```python
from build123d import *

# Parameters (mm, degrees)
F0_W     = 62
F0_H     = 82
F0_R     = 9.1
F1_DEPTH = 2
F2_R     = 10
F3_R     = 10
F4_R     = 10
F5_R     = 10
F7_DEPTH = 1


with BuildPart() as f1:
    # F0 (on Right) → F1 (new body)
    with BuildSketch(Plane.YZ):
        with Locations((0, -10)):
            Rectangle(F0_W, F0_H)
        with Locations((-20, -40)):
            Circle(F0_R, mode=Mode.SUBTRACT)
        with Locations((-20, -20)):
            Circle(F0_R, mode=Mode.SUBTRACT)
        with Locations((0, -40)):
            Circle(F0_R, mode=Mode.SUBTRACT)
        with Locations((20, -40)):
            Circle(F0_R, mode=Mode.SUBTRACT)
        with Locations((0, -20)):
            Circle(F0_R, mode=Mode.SUBTRACT)
        with Locations((20, -20)):
            Circle(F0_R, mode=Mode.SUBTRACT)
        with Locations((-20, 0)):
            Circle(F0_R, mode=Mode.SUBTRACT)
        with Locations((-20, 20)):
            Circle(F0_R, mode=Mode.SUBTRACT)
        Circle(F0_R, mode=Mode.SUBTRACT)
        with Locations((20, 0)):
            Circle(F0_R, mode=Mode.SUBTRACT)
        with Locations((0, 20)):
            Circle(F0_R, mode=Mode.SUBTRACT)
        with Locations((20, 20)):
            Circle(F0_R, mode=Mode.SUBTRACT)
    extrude(amount=F1_DEPTH)

    # F2
    f2_edges = [f1.edges().sort_by_distance(p)[0] for p in [
        (1, 31, 31),
    ]]
    fillet(f2_edges, radius=F2_R)

    # F3
    f3_edges = [f1.edges().sort_by_distance(p)[0] for p in [
        (1, -31, 31),
    ]]
    fillet(f3_edges, radius=F3_R)

    # F4
    f4_edges = [f1.edges().sort_by_distance(p)[0] for p in [
        (1, 31, -51),
    ]]
    fillet(f4_edges, radius=F4_R)

    # F5
    f5_edges = [f1.edges().sort_by_distance(p)[0] for p in [
        (1, -31, -51),
    ]]
    fillet(f5_edges, radius=F5_R)

    # F6 (on face) → F7 (join)
    with BuildSketch(Plane.YZ.offset(2)):
        with BuildLine():
            ThreePointArc((-31, -41), (-28.071068, -48.071068), (-21, -51))
            Line((-21, -51), (21, -51))
            ThreePointArc((21, -51), (28.071068, -48.071068), (31, -41))
            Line((31, -41), (31, 21))
            ThreePointArc((31, 21), (28.071068, 28.071068), (21, 31))
            Line((21, 31), (-21, 31))
            ThreePointArc((-21, 31), (-28.071068, 28.071068), (-31, 21))
            Line((-31, 21), (-31, -41))
        make_face()
        with BuildLine():
            ThreePointArc((-29.5, 21), (-27.010408, 27.010408), (-21, 29.5))
            Line((-21, 29.5), (21, 29.5))
            ThreePointArc((21, 29.5), (27.010408, 27.010408), (29.5, 21))
            Line((29.5, 21), (29.5, -41))
            ThreePointArc((29.5, -41), (27.010408, -47.010408), (21, -49.5))
            Line((21, -49.5), (-21, -49.5))
            ThreePointArc((-21, -49.5), (-27.010408, -47.010408), (-29.5, -41))
            Line((-29.5, -41), (-29.5, 21))
        make_face(mode=Mode.SUBTRACT)
    extrude(amount=F7_DEPTH)


solid = f1.part
```
Could you check a few things on this model? Use its own coordinates, in mm. A direction names the side the tool comes from. Round coordinates to 2 decimals unless told otherwise and drop trailing zeros. Order: outer loops, then holes, each group sorted by start corner. A loop starts at its lowest first (then second) coordinate and runs counter-clockwise, first axis right, second up. Notation, with made-up numbers: (-20, 31) -> (14, 31) arc R34 cw to (14, 66) -> close; hole circle Ø11 at (38.5, -39.75). An arc over 180 degrees is marked (long way). One line per question, with ' | ' between items.
Q1. If we section it at C-C on x = 0.6: Give the number of separate pieces and of enclosed holes in the cut face, plus the area to 3 significant figures.
Computed values:
separate pieces: 1 | enclosed holes: 12 | area: 1,880 mm²
Q2. I'm going to push a flat-ended pin straight in: pin 1 (16.5 mm diameter, centred on y = 0, z = -20, fed in from +X). Where does the tip first touch, or does it pass through?
Computed values:
pin 1: through
Q3. We'd pull the mould along Z, two halves only. Please class faces 3 (the face through (0.986, 24.892, -32.327)), 4 (the face through (1, 31, -10)), 5 (the face through (1, 0, -51)): released by +Z, released by -Z, zero draft, split by the parting line, or undercut.
Computed values:
face 3: undercut | face 4: zero draft | face 5: released by -Z
Q4. If I drill on line 1 (Z direction, x = 1.55, y = -20); line 2 (Y direction, x = 1.1, z = 6.5); line 3 (Z direction, x = 0.65, y = 13), over which ranges is the centre line in solid material (lowest first)? Write a range as from..to.
Computed values:
line 1: -51..-49.1, -30.9..-29.1, -10.9..-9.1, 9.1..10.9, 29.1..31 | line 2: -31..-26.37, -13.63..-6.37, 6.37..13.63, 26.37..31 | line 3: -51..-45.81, -34.19..-25.81, -14.19..-5.81, 5.81..14.19, 25.81..31
Q5. If we section it at A-A on z = 20: Write out the boundary of the cut face in (x, y).
Computed values:
outline: (0, -31) -> (3, -31) -> (3, -29.5) -> (2, -29.5) -> (2, -29.1) -> (0, -29.1) -> close; (0, -10.9) -> (2, -10.9) -> (2, -9.1) -> (0, -9.1) -> close; (0, 9.1) -> (2, 9.1) -> (2, 10.9) -> (0, 10.9) -> close; (0, 29.1) -> (2, 29.1) -> (2, 29.5) -> (3, 29.5) -> (3, 31) -> (0, 31) -> close
Q6. Which directions (+Z, -Z, +X, -X, +Y, -Y) give clear straight access to the entire face, cutting with the end or side of a thin tool? Please do faces 1 (the face through (0.986, -1.973, 11.116)), 2 (the face through (2.49, -27.08, 26.94)).
Computed values:
face 1: +X, -X | face 2: +X
Q7. If we section it at D-D on y = -20: Write out the boundary of the cut face in (x, z), plus the area to 3 significant figures.
Computed values:
outline: (0, -51) -> (3, -51) -> (3, -49.5) -> (2, -49.5) -> (2, -49.1) -> (0, -49.1) -> close; (0, -30.9) -> (2, -30.9) -> (2, -29.1) -> (0, -29.1) -> close; (0, -10.9) -> (2, -10.9) -> (2, -9.1) -> (0, -9.1) -> close; (0, 9.1) -> (2, 9.1) -> (2, 10.9) -> (0, 10.9) -> close; (0, 29.1) -> (2, 29.1) -> (2, 29.5) -> (3, 29.5) -> (3, 31) -> (0, 31) -> close | area: 21.4 mm²
Q8. If we section it at B-B on y = 3.5: Write out the boundary of the cut face in (x, z), plus the area to 3 significant figures.
Computed values:
outline: (0, -51) -> (3, -51) -> (3, -49.5) -> (2, -49.5) -> (2, -48.4) -> (0, -48.4) -> close; (0, -31.6) -> (2, -31.6) -> (2, -28.4) -> (0, -28.4) -> close; (0, -11.6) -> (2, -11.6) -> (2, -8.4) -> (0, -8.4) -> close; (0, 8.4) -> (2, 8.4) -> (2, 11.6) -> (0, 11.6) -> close; (0, 28.4) -> (2, 28.4) -> (2, 29.5) -> (3, 29.5) -> (3, 31) -> (0, 31) -> close | area: 32.6 mm²
